Build history of the part. All positions in model axes, mm. Face numbers are marked on the shaded views. Round coordinates to 2 decimals unless told otherwise and drop trailing zeros. Order: outer loops, then holes, each group sorted by start corner. A loop starts at its lowest first (then second) coordinate and runs counter-clockwise, first axis right, second up. Notation, with made-up numbers: (-1, -11) -> (34, -11) arc R38 cw to (34, 28) -> close; hole circle Ø5 at (-32, 32). An arc over 180 degrees is marked (long way). Answer as CSV lines item,"result". Start each with the question number.
```python
from build123d import *

# Parameters (mm, degrees)
CROQUIS1_R              = 59.5
SALIENTE_EXTRUIR1_DEPTH = 53
CROQUIS2_R              = 40
SALIENTE_EXTRUIR2_DEPTH = 8.5
CORTAR_EXTRUIR1_REACH   = 106.225
CROQUIS4_R              = 30
CROQUIS5_R              = 0.65
SALIENTE_EXTRUIR3_DEPTH = 10
CROQUIS6_R              = 0.65
SALIENTE_EXTRUIR4_DEPTH = 10
SALIENTE_EXTRUIR5_DEPTH = 4


with BuildPart() as part:
    # Croquis1 → Saliente-Extruir1 (new body)
    with BuildSketch(Plane(origin=(0, 0, 0), x_dir=(1, 0, 0), z_dir=(0, 1, 0))):
        with Locations(Location((0, 0, 0), (0, 0, 270))):
            Circle(CROQUIS1_R)
    extrude(amount=SALIENTE_EXTRUIR1_DEPTH)

    # Croquis2 → Saliente-Extruir2 (add)
    with BuildSketch(Plane(origin=(0, 53, 0), x_dir=(1, 0, 0), z_dir=(0, 1, 0))):
        with Locations(Location((0, 0, 0), (0, 0, 270))):
            Circle(CROQUIS2_R)
    extrude(amount=SALIENTE_EXTRUIR2_DEPTH)

    # Croquis4 → Cortar-Extruir1 (cut, up to next)
    with BuildSketch(Plane(origin=(0, 61.5, 0), x_dir=(1, 0, 0), z_dir=(0, 1, 0)), mode=Mode.PRIVATE) as cortar_extruir1_sk1:
        with Locations(Location((0, 0, 0), (0, 0, 270))):
            Circle(CROQUIS4_R)
    cortar_extruir1_tool1 = extrude(cortar_extruir1_sk1.sketch, amount=-CORTAR_EXTRUIR1_REACH, mode=Mode.PRIVATE) & part.part
    add(cortar_extruir1_tool1.solids().sort_by_distance((0, 61.5, 0))[0], mode=Mode.SUBTRACT)

    # Croquis5 → Saliente-Extruir3 (add)
    with BuildSketch(Plane(origin=(0, 61.5, 0), x_dir=(1, 0, 0), z_dir=(0, 1, 0))):
        with Locations(Location((35, 0, 0), (0, 0, 270))):
            Circle(CROQUIS5_R)
        with Locations(Location((34.866814433, 3.050450996, 0), (0, 0, 270))):
            Circle(CROQUIS5_R)
        with Locations(Location((34.866814433, -3.050450996, 0), (0, 0, 90))):
            Circle(CROQUIS5_R)
    extrude(amount=SALIENTE_EXTRUIR3_DEPTH)

    # Croquis6 → Saliente-Extruir4 (add)
    with BuildSketch(Plane.XZ):
        with Locations(Location((45, 0, 0), (0, 0, 90))):
            Circle(CROQUIS6_R)
        with Locations(Location((44.828761414, 3.922008424, 0), (0, 0, 90))):
            Circle(CROQUIS6_R)
        with Locations(Location((44.828761414, -3.922008424, 0), (0, 0, 90))):
            Circle(CROQUIS6_R)
    extrude(amount=SALIENTE_EXTRUIR4_DEPTH)

    # Croquis10 → Saliente-Extruir5 (add)
    with BuildSketch(Plane.XZ):
        with BuildLine():
            ThreePointArc((4.75, 68), (0, 63.25), (-4.75, 68))
            Line((-4.75, 68), (-4.75, 78))
            Line((-4.75, 78), (-9.75, 78))
            Line((-9.75, 78), (-9.75, 48))
            Line((-9.75, 48), (9.75, 48))
            Line((9.75, 48), (9.75, 78))
            Line((9.75, 78), (4.75, 78))
            Line((4.75, 78), (4.75, 68))
        make_face()
    extrude(amount=SALIENTE_EXTRUIR5_DEPTH)


solid = part.part
```
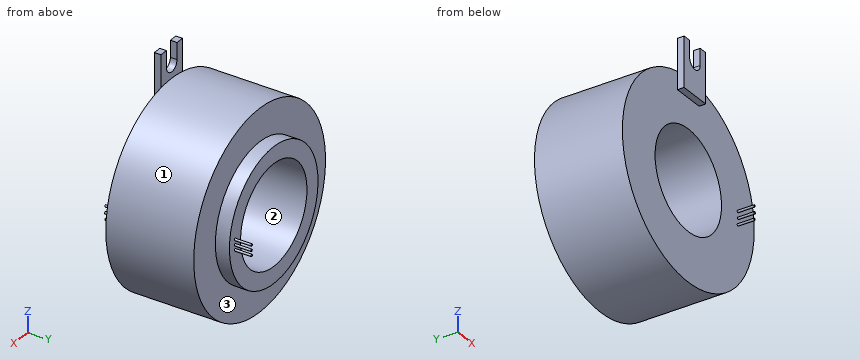
Q1. Slice it at D-D, the plane x = 0. Write the cut outline in (y, z), plus the area to 3 significant figures.
Q2. Probe L1, parallel to X at y = 40, z = 0; L2, parallel to Y at x = -25, z = -44; L3, parallel to Y at x = 31.5, z = 23. List the from-to ranges inside material, lowest first.
Q3. Slice it at B-B, the plane z = -19.5. Write the cut outline in (x, y), plus the area to 3 significant figures.
Q4. Slice it at A-A, the plane x = -27.5. Write the cut outline in (y, z), plus the area to 3 significant figures.
Q5. Two-plate mould, pull along Z, no slides. Class the marked faces 1, 2 and 3: +Z half, -Z half, draft (parallel to the pull), parting line (faces both ways), or undercut.
Q6. Flat gauge pins, fed straight in: pin 1 Ø6 at (y, z) = (34.5, 21) entering from -X; pin 2 Ø1.5 at (x, y) = (33.5, 31) entering from +Z; pin 3 Ø6 at (y, z) = (29.5, -1.5) entering from -X. Where does each tip first touch, or does it go through?
Q7. Slice it at C-C, the plane y = 43. Write the cut outline in (x, z).
Solutions:
1,outline,"(-4, 48) -> (0, 48) -> (0, 30) -> (61.5, 30) -> (61.5, 40) -> (53, 40) -> (53, 59.5) -> (0, 59.5) -> (0, 63.25) -> (-4, 63.25) -> close; (0, -59.5) -> (53, -59.5) -> (53, -40) -> (61.5, -40) -> (61.5, -30) -> (0, -30) -> close"
1,area,"3,360 mm2"
2,L1,"x = -59.5 to -30, 30 to 59.5"
2,L2,"y = 0 to 53"
2,L3,"y = 0 to 61.5"
3,outline,"(-56.21, 0) -> (-22.8, 0) -> (-22.8, 61.5) -> (-34.92, 61.5) -> (-34.92, 53) -> (-56.21, 53) -> close; (22.8, 0) -> (56.21, 0) -> (56.21, 53) -> (34.92, 53) -> (34.92, 61.5) -> (22.8, 61.5) -> close"
3,area,"3,750 mm2"
4,outline,"(0, -52.76) -> (53, -52.76) -> (53, -29.05) -> (61.5, -29.05) -> (61.5, -11.99) -> (0, -11.99) -> close; (0, 11.99) -> (61.5, 11.99) -> (61.5, 29.05) -> (53, 29.05) -> (53, 52.76) -> (0, 52.76) -> close"
4,area,"4,610 mm2"
5,face 1,"parting line"
5,face 2,"undercut"
5,face 3,"draft"
6,pin 1,"stops at x = -56.71"
6,pin 2,"stops at z = 49.68"
6,pin 3,"stops at x = -59.5"
7,outline,"circle Ø119 at (0, 0); hole circle Ø60 at (0, 0)"
